```python
from build123d import *

# Parameters (mm, degrees)
SKETCH_1_R          = 13
EXTRUDE_1_DEPTH     = 20
SKETCH_2_R          = 13
EXTRUDE_2_DEPTH     = 400
SKETCH_4_W          = 140
SKETCH_4_H          = 85
EXTRUDE_3_DEPTH     = 210
SHELL_2_T           = -5
SKETCH_5_W          = 130
SKETCH_5_H          = 5
CUT_EXTRUDE_3_DEPTH = 80
SKETCH_6_R          = 30
SKETCH_6_R_2        = 3.25
CUT_EXTRUDE_4_DEPTH = 10
SKETCH_3_R          = 11
CUT_EXTRUDE_5_DEPTH = 425
SKETCH_7_R          = 13
CUT_EXTRUDE_6_DEPTH = 420
SKETCH_8_R          = 2.5
CUT_EXTRUDE_7_DEPTH = 5


with BuildPart() as part:
    # 草图1 → 凸台-拉伸1 (new body)
    with BuildSketch(Plane(origin=(0, 0, 0), x_dir=(1, 0, 0), z_dir=(0, 1, 0))):
        Circle(SKETCH_1_R)
    extrude(amount=EXTRUDE_1_DEPTH)

    # 草图2 → 凸台-拉伸2 (add)
    with BuildSketch(Plane(origin=(0, 20, 0), x_dir=(1, 0, 0), z_dir=(0, 1, 0))):
        Circle(SKETCH_2_R)
    extrude(amount=EXTRUDE_2_DEPTH)


with BuildPart() as body_2:
    # 草图4 → 凸台-拉伸3 (new body)
    with BuildSketch(Plane.XZ):
        with Locations((0, -20)):
            Rectangle(SKETCH_4_W, SKETCH_4_H)
    extrude(amount=EXTRUDE_3_DEPTH)

    # 抽壳2
    shell_2_openings = [body_2.faces().sort_by_distance(p)[0] for p in [
        (0, -105, 22.5),
    ]]
    offset(amount=SHELL_2_T, openings=shell_2_openings, kind=Kind.INTERSECTION)

    # 草图5 → 切除-拉伸3 (cut)
    with BuildSketch(Plane.XY.offset(22.5)):
        with Locations((0, -207.5)):
            Rectangle(SKETCH_5_W, SKETCH_5_H)
    extrude(amount=-CUT_EXTRUDE_3_DEPTH, mode=Mode.SUBTRACT)

    # 草图6 → 切除-拉伸4 (cut)
    with BuildSketch(Plane(origin=(0, 0, -62.5), x_dir=(-1, 0, 0), z_dir=(0, 0, -1))):
        with Locations((0, -150)):
            Circle(SKETCH_6_R)
        with Locations((26.516504294, -123.483495706)):
            Circle(SKETCH_6_R_2)
        with Locations((26.516504294, -176.516504294)):
            Circle(SKETCH_6_R_2)
        with Locations((-26.516504294, -176.516504294)):
            Circle(SKETCH_6_R_2)
        with Locations((-26.516504294, -123.483495706)):
            Circle(SKETCH_6_R_2)
    extrude(amount=-CUT_EXTRUDE_4_DEPTH, mode=Mode.SUBTRACT)


with BuildPart() as cut_extrude_5_tool:
    # 草图3 → 切除-拉伸5 (new body)
    with BuildSketch(Plane(origin=(0, 420, 0), x_dir=(1, 0, 0), z_dir=(0, 1, 0))):
        Circle(SKETCH_3_R)
    extrude(amount=-CUT_EXTRUDE_5_DEPTH)


with BuildPart() as part_1:
    add(part.part)

    # 切除-拉伸5: cut by cut_extrude_5_tool
    add(cut_extrude_5_tool.part, mode=Mode.SUBTRACT)

    # 草图7 → 切除-拉伸6 (cut)
    with BuildSketch(Plane(origin=(0, 420, 0), x_dir=(1, 0, 0), z_dir=(0, 1, 0))):
        Circle(SKETCH_7_R)
    extrude(amount=-CUT_EXTRUDE_6_DEPTH, mode=Mode.SUBTRACT)


with BuildPart() as body_2_1:
    add(body_2.part)

    # 切除-拉伸5: cut by cut_extrude_5_tool
    add(cut_extrude_5_tool.part, mode=Mode.SUBTRACT)

    # 草图8 → 切除-拉伸7 (cut)
    with BuildSketch(Plane(origin=(0, 0, 0), x_dir=(1, 0, 0), z_dir=(0, 1, 0))):
        with Locations((-32.020865922, -16.5)):
            Circle(SKETCH_8_R)
        with Locations((-32.020865922, 18.5)):
            Circle(SKETCH_8_R)
        with Locations((31.979134078, -16.5)):
            Circle(SKETCH_8_R)
        with Locations((31.979134078, 18.5)):
            Circle(SKETCH_8_R)
    extrude(amount=-CUT_EXTRUDE_7_DEPTH, mode=Mode.SUBTRACT)


solid = body_2_1.part
```
Here's how the part is built. I have some questions about the finished solid (model axes, mm). A direction names the side the tool comes from. Give positions to 0.01 mm unless a question says otherwise; leave off trailing zeros. Write each loop counter-clockwise with the first axis right and the second up, starting at its lowest first coordinate (ties: lowest second). Pieces come first, ordered by that corner, then holes. Notation, with made-up numbers: M -22,-29 L 31,-29 A4 ccw 31,-22 Z; hole C 5,-5 d1. An arc over 180 degrees is marked long. Put each result on its own line as item: value. Start each with the question number.
Item 1: If we section it at D-D, the plane x = -21: Write out the boundary of the cut face in (y, z), then the cut area to 3 significant figures.
Item 2: Will these pins go through, and if not, where does the flat tip stop? pin 1 (8 mm diameter, centred on x = -32.02, z = -18.5, fed in from -Y); pin 2 (8.5 mm diameter, centred on x = -26.52, y = -176.52, fed in from +Z); pin 3 (5 mm diameter, centred on x = -26.52, y = -123.48, fed in from +Z); pin 4 (8.5 mm diameter, centred on x = 26.52, y = -176.52, fed in from -Z).
Item 3: Thinking about a two-plate mould opening in Z: for faces 3 (the flat face through (-1, -104, -62.5)), 4 (the cylindrical face through (-2.38, -2.46, 10.74)), 5 (the cylindrical face through (30.137, -2.465, -20.19)), 6 (the cylindrical face through (27.221, -126.656, -60.035)), which applies, +Z half, -Z half, draft (parallel to the pull), parting line (faces both ways), or undercut?
Item 4: I need wall thicknesses on L1, parallel to X at y = -2, z = -18; L2, parallel to X at y = -109, z = -39.5; L3, parallel to Y at x = 0, z = -60. Which ranges of each line are inside material? Lowest first, please. Write a range as from..to.
Item 5: If we section it at A-A, the plane x = 0: Write out the boundary of the cut face in (y, z), then the cut area to 3 significant figures.
Item 6: If we section it at B-B, the plane y = -150: Write out the boundary of the cut face in (x, z), then the cut area to 3 significant figures.
Item 7: On a 3-axis mill with a long thin cutter (end or side, diameter ignored), from which of +Z, -Z, +X, -X, +Y, -Y can I reach the whole of each face in a straight line? I mean faces 1 (the flat face through (-1, -106, -57.5)), 2 (the cylindrical face through (-32, -2, -21)). Say none if no direction works.
Item 8: If we section it at C-C, the plane z = 16.5: Write out the boundary of the cut face in (x, y), then the cut area to 3 significant figures.
Values:
1. outline: M -210,-62.5 L -171.42,-62.5 L -171.42,-57.5 L -210,-57.5 Z; M -128.58,-62.5 L 0,-62.5 L 0,22.5 L -5,22.5 L -5,-57.5 L -128.58,-57.5 Z
1. area: 1,240 mm²
2. pin 1: y = -5
2. pin 2: z = -57.5
2. pin 3: through
2. pin 4: z = -62.5
3. face 3: -Z half
3. face 4: undercut
3. face 5: undercut
3. face 6: draft
4. L1: -70..-34.47, -29.57..29.53, 34.43..70
4. L2: -70..-65, 65..70
4. L3: -210..-180, -120..0
5. outline: M -210,-62.5 L -180,-62.5 L -180,-57.5 L -210,-57.5 Z; M -120,-62.5 L 0,-62.5 L 0,-11 L -5,-11 L -5,-57.5 L -120,-57.5 Z; M -5,11 L 0,11 L 0,22.5 L -5,22.5 Z
5. area: 1,040 mm²
6. outline: M -70,-62.5 L -30,-62.5 L -30,-57.5 L -65,-57.5 L -65,22.5 L -70,22.5 Z; M 30,-62.5 L 70,-62.5 L 70,22.5 L 65,22.5 L 65,-57.5 L 30,-57.5 Z
6. area: 1,200 mm²
7. face 1: +Z, -Y
7. face 2: +Y, -Y
8. outline: M -70,-210 L -65,-210 L -65,-5 L -34.52,-5 L -34.52,0 L -70,0 Z; M -29.52,-5 L 29.48,-5 L 29.48,0 L -29.52,0 Z; M 34.48,-5 L 65,-5 L 65,-210 L 70,-210 L 70,0 L 34.48,0 Z
8. area: 2,700 mm²
